Design review of the part built by this model. Coordinates are the model's own, in mm. Give positions to 0.01 mm unless a question says otherwise; leave off trailing zeros. Loops run counter-clockwise (first coordinate to the right, second up) from the corner with the lowest first, then second, coordinate; pieces in that order, holes last. Notation, with made-up numbers: (12, 13.25) - (68, 13.25) arc R20 ccw to (68, 33.25) - close; hole circle Ø7 at (34.25, 27.25). An arc over 180 degrees is marked (long way). Write each question's results on one line, items separated by ' | '.
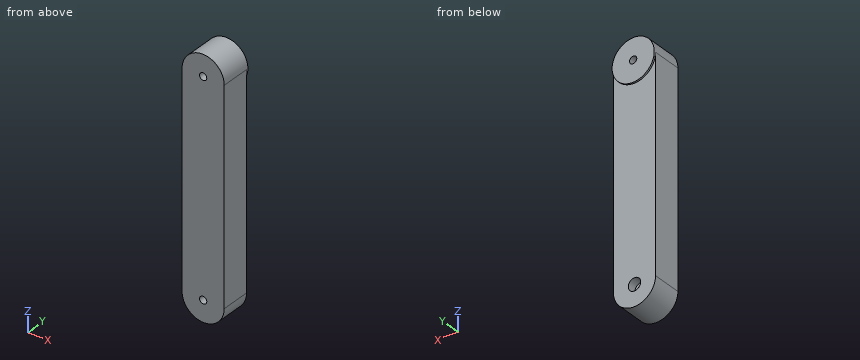
from build123d import *

# Parameters (mm, degrees)
SKETCH1_R           = 2.05
BOSS_EXTRUDE1_DEPTH = 17.7
SKETCH2_R           = 3.55
CUT_EXTRUDE1_DEPTH  = 6
CUT_EXTRUDE2_START  = -1
CUT_EXTRUDE2_DEPTH  = 1


with BuildPart() as part:
    # Sketch1 → Boss-Extrude1 (new body)
    with BuildSketch(Plane(origin=(0, 0, 0), x_dir=(1, 0, 0), z_dir=(0, 1, 0))):
        with BuildLine():
            Line((-12, -60), (-12, 60))
            ThreePointArc((-12, 60), (0, 72), (12, 60))
            Line((12, 60), (12, -60))
            ThreePointArc((12, -60), (0, -72), (-12, -60))
        make_face()
        with Locations(Location((0, 60, 0), (0, 0, 270))):
            Circle(SKETCH1_R, mode=Mode.SUBTRACT)
        with Locations(Location((0, -60, 0), (0, 0, 270))):
            Circle(SKETCH1_R, mode=Mode.SUBTRACT)
    extrude(amount=BOSS_EXTRUDE1_DEPTH)

    # Sketch2 → Cut-Extrude1 (cut)
    with BuildSketch(Plane(origin=(0, 17.7, 0), x_dir=(1, 0, 0), z_dir=(0, 1, 0))):
        with Locations(Location((0, 60, 0), (0, 0, 270))):
            Circle(SKETCH2_R)
    extrude(amount=-CUT_EXTRUDE1_DEPTH, mode=Mode.SUBTRACT)

    # Sketch3 → Cut-Extrude2 (cut)
    with BuildSketch(Plane(origin=(0, 17.7, 0), x_dir=(1, 0, 0), z_dir=(0, 1, 0)).offset(CUT_EXTRUDE2_START)):
        with BuildLine():
            Line((12, -60), (12, 60))
            ThreePointArc((12, 60), (0, 72), (-12, 60))
            Line((-12, 60), (-12, -60))
            ThreePointArc((-12, -60), (0, -48), (12, -60))
        make_face()
    extrude(amount=CUT_EXTRUDE2_DEPTH, mode=Mode.SUBTRACT)


solid = part.part
(1) Wall thickness on line 1 along Z through (x, y) = (0.75, 13.5); line 2 along X through (y, z) = (12.9, -60); line 3 along X through (y, z) = (5.25, -60): over which ranges is each line inside the solid? List them lowest first. Write a range as from..to.
Answers below:
line 1: -71.98..-63.47, -56.53..58.09, 61.91..71.98 | line 2: -12..-3.55, 3.55..12 | line 3: -12..-2.05, 2.05..12
(2) Take a section at A-A on x = 0. Give the boundary of the cut face in (y, z), plus the area to 3 significant figures.
Answers below:
outline: (0, -72) - (16.7, -72) - (16.7, -63.55) - (11.7, -63.55) - (11.7, -62.05) - (0, -62.05) - close; (0, -57.95) - (11.7, -57.95) - (11.7, -56.45) - (16.7, -56.45) - (16.7, 48) - (17.7, 48) - (17.7, 57.95) - (0, 57.95) - close; (0, 62.05) - (17.7, 62.05) - (17.7, 72) - (0, 72) - close | area: 2,270 mm2
(3) Take a section at C-C on z = -36.5. Give the boundary of the cut face in (x, y), plus the area to 3 significant figures.
Answers below:
outline: (-12, 0) - (12, 0) - (12, 16.7) - (-12, 16.7) - close | area: 401 mm2
(4) Insertion check: P1, Ø6, axis at x = 9.5, z = -44, coming from the +Y side; P2, Ø2, axis at x = -1.5, z = -59.5, coming from the +Y side; P3, Ø1.5, axis at x = -9, y = 11, coming from the -Z side. Each pin has a flat end and moves straight along its axis. Give the tip position at first contact, or say it passes through.
Answers below:
P1: y = 16.7 | P2: y = 11.7 | P3: z = -68.71
(5) Take a section at B-B on y = 13. Give the boundary of the cut face in (x, z).
Answers below:
outline: (-12, -60) arc R12 ccw to (12, -60) - (12, 60) arc R12 ccw to (-12, 60) - close; hole circle Ø7.1 at (0, -60); hole circle Ø4.1 at (0, 60)
(6) Take a section at D-D on x = 8.25. Give the boundary of the cut face in (y, z), plus the area to 3 significant figures.
Answers below:
outline: (0, -68.71) - (16.7, -68.71) - (16.7, 51.29) - (17.7, 51.29) - (17.7, 68.71) - (0, 68.71) - close | area: 2,310 mm2
